from build123d import *

# Parameters (mm, degrees)
SKETCH1_W                 = 23
SKETCH1_H                 = 18.6
BOSS_EXTRUDE1_DEPTH       = 4.8
SKETCH2_W                 = 15.1
SKETCH2_H                 = 2.7
CUT_EXTRUDE1_DEPTH        = 27.8
SKETCH3_W                 = 12
SKETCH3_H                 = 10
CUT_EXTRUDE2_DEPTH        = 27.8
M2X0_4_TAPPED_HOLE1_D     = 1.6
M2X0_4_TAPPED_HOLE1_DEPTH = 4
M2X0_4_TAPPED_HOLE1_TIP   = 0.480688495
SKETCH7_R                 = 1.3
CUT_EXTRUDE3_DEPTH        = 27.8
FILLET1_R                 = 1


with BuildPart() as part:
    # Sketch1 → Boss-Extrude1 (new body)
    with BuildSketch(Plane(origin=(0, 0, 0), x_dir=(1, 0, 0), z_dir=(0, 1, 0))):
        Rectangle(SKETCH1_W, SKETCH1_H)
    extrude(amount=BOSS_EXTRUDE1_DEPTH)

    # Sketch2 → Cut-Extrude1 (cut)
    with BuildSketch(Plane(origin=(11.5, 0, 0), x_dir=(0, 0, -1), z_dir=(1, 0, 0))):
        with Locations((-1.75, 3.45)):
            Rectangle(SKETCH2_W, SKETCH2_H)
    extrude(amount=-CUT_EXTRUDE1_DEPTH, mode=Mode.SUBTRACT)

    # Sketch3 → Cut-Extrude2 (cut)
    with BuildSketch(Plane.XZ):
        with Locations((0, -4.3)):
            Rectangle(SKETCH3_W, SKETCH3_H)
    extrude(amount=-CUT_EXTRUDE2_DEPTH, mode=Mode.SUBTRACT)

    # M2x0.4 Tapped Hole1
    with Locations(Plane(origin=(0, 0, -9.3), x_dir=(-1, 0, 0), z_dir=(0, 0, -1))):
        with Locations((-8.5, 2.2), (8.5, 2.2)):
            Hole(M2X0_4_TAPPED_HOLE1_D / 2, depth=M2X0_4_TAPPED_HOLE1_DEPTH)
            with Locations((0, 0, -(M2X0_4_TAPPED_HOLE1_DEPTH + M2X0_4_TAPPED_HOLE1_TIP / 2))):  # 118° drill point
                Cone(0, M2X0_4_TAPPED_HOLE1_D / 2, M2X0_4_TAPPED_HOLE1_TIP, mode=Mode.SUBTRACT)

    # Sketch7 → Cut-Extrude3 (cut)
    with BuildSketch(Plane.XZ):
        with Locations((-8.5, 6.7)):
            Circle(SKETCH7_R)
        with Locations((8.5, 6.7)):
            Circle(SKETCH7_R)
    extrude(amount=-CUT_EXTRUDE3_DEPTH, mode=Mode.SUBTRACT)

    # Fillet1
    fillet1_edges = [part.edges().sort_by_distance(p)[0] for p in [
        (-6, 1.05, 0.7),
        (6, 1.05, 0.7),
    ]]
    fillet(fillet1_edges, radius=FILLET1_R)


solid = part.part
For this review, take the finished solid that the model builds, in its own axes (mm). A direction names the side the tool comes from. Give positions to 0.01 mm unless a question says otherwise; leave off trailing zeros. Write each loop counter-clockwise with the first axis right and the second up, starting at its lowest first coordinate (ties: lowest second). Pieces come first, ordered by that corner, then holes. Notation, with made-up numbers: (74, 81) -> (111, 81) arc R26 cw to (111, 110) -> close; hole circle Ø6 at (12.25, 31.25). An arc over 180 degrees is marked (long way). Use CSV: the item, a comma, the result in double quotes.
Q1. Take a section at B-B, the plane z = 6.7. Write out the cut boundary in (x, y).
Conclusion:
outline,"(-11.5, 0) -> (-9.8, 0) -> (-9.8, 2.1) -> (-11.5, 2.1) -> close; (-7.2, 0) -> (7.2, 0) -> (7.2, 2.1) -> (-7.2, 2.1) -> close; (9.8, 0) -> (11.5, 0) -> (11.5, 2.1) -> (9.8, 2.1) -> close"
Q2. Take a section at A-A, the plane z = -6.75. Write out the cut boundary in (x, y).
Conclusion:
outline,"(-11.5, 0) -> (-6, 0) -> (-6, 4.8) -> (-11.5, 4.8) -> close; (6, 0) -> (11.5, 0) -> (11.5, 4.8) -> (6, 4.8) -> close; hole circle Ø1.6 at (-8.5, 2.2); hole circle Ø1.6 at (8.5, 2.2)"
Q3. To check wall thickness, follow probe 1 along X at (y, z) = (2.25, -7); probe 2 along X at (y, z) = (0.6, -3.5); probe 3 along Z at (x, y) = (8.5, 0.9). State the ranges of each line that lie inside material, in increasing order. Write a range as [from, to].
Conclusion:
probe 1,"[-11.5, -9.3], [-7.7, -6], [6, 7.7], [9.3, 11.5]"
probe 2,"[-11.5, -6], [6, 11.5]"
probe 3,"[-9.3, 5.4], [8, 9.3]"
Q4. Tool access review of faces 1 (the face through (5.699, 1.065, 0.415)), 2 (the face through (-8.7, 3.4, -5.8)), 3 (the face through (8.33, 1.42, -7.27)): name each direction out of +Z, -Z, +X, -X, +Y, -Y from which nothing blocks a thin tool from reaching the whole face with its end or side.
Conclusion:
face 1,"-Z, +Y, -Y"
face 2,"+Z, +X, -X, +Y"
face 3,"-Z"
Q5. Take a section at C-C, the plane x = -8.5. Write out the cut boundary in (y, z).
Conclusion:
outline,"(0, -9.3) -> (1.4, -9.3) -> (1.4, -5.3) -> (2.1, -4.88) -> (2.1, 5.4) -> (0, 5.4) -> close; (0, 8) -> (2.1, 8) -> (2.1, 9.3) -> (0, 9.3) -> close; (3, -9.3) -> (4.8, -9.3) -> (4.8, -5.8) -> (3, -5.8) -> close"
Q6. Mouldability with a two-part tool opening along X and no side actions: class faces 4 (the face through (-9, 4.8, -8)), 5 (the face through (11.5, 1, -2)), 6 (the face through (-6, 2, -6)) as pulls with the +X half, pulls with the -X half, needs draft (parallel to the pull), parting line crosses it, or undercut.
Conclusion:
face 4,"needs draft"
face 5,"pulls with the +X half"
face 6,"undercut"
Q7. For P1, Ø2.5, axis at x = 8.5, y = 2.2, coming from the +Z side; P2, Ø2.5, axis at x = -0.5, y = 1, coming from the -Z side; P3, Ø2, axis at x = 8.5, z = 6.7, coming from the -Y side; P4, Ø1.4, axis at x = 10, y = 4, coming from the +Z side, all flat-tipped, find the tip position at first contact; note any pin that passes through.
Conclusion:
P1,"z = 9.3"
P2,"z = 0.7"
P3,"through"
P4,"z = -5.8"
Q8. Take a section at D-D, the plane y = 1. Write out the cut boundary in (x, z).
Conclusion:
outline,"(-11.5, -9.3) -> (-6, -9.3) -> (-6, -0.3) arc R1 cw to (-5, 0.7) -> (5, 0.7) arc R1 cw to (6, -0.3) -> (6, -9.3) -> (11.5, -9.3) -> (11.5, 9.3) -> (-11.5, 9.3) -> close; hole circle Ø2.6 at (-8.5, 6.7); hole circle Ø2.6 at (8.5, 6.7)"
